from build123d import *

# Parameters (mm, degrees)
CYLINDER055_R       = 2.5
CYLINDER055_DEPTH   = 100
ARRAY001032_Y_COUNT = 6
ARRAY001032_Y_PITCH = 50
BOX030_W            = 3
BOX030_H            = 280
BOX030_DEPTH        = 20
FILLET002_R         = 4


with BuildPart() as horizontal_hole_array006:
    # Cylinder055 → Cylinder055 (new body)
    with BuildSketch(Plane(origin=(-137, -85, -101), x_dir=(0, 0, -1), z_dir=(1, 0, 0))):
        Circle(CYLINDER055_R)
    extrude(amount=CYLINDER055_DEPTH)

    # Array001032 Y: horizontal hole array006 ×6


with BuildPart() as horizontal_hole_array006_1:
    add(horizontal_hole_array006.part)
    with Locations(*[(0, i * ARRAY001032_Y_PITCH, 0) for i in range(1, ARRAY001032_Y_COUNT)]):
        add(horizontal_hole_array006.part)


with BuildPart() as stand_attachment_bottom_plate_cut:
    # Box030 → Box030 (new body)
    with BuildSketch(Plane(origin=(-103, -100, -111), x_dir=(1, 0, 0), z_dir=(0, 0, 1))):
        with Locations((1.5, 140)):
            Rectangle(BOX030_W, BOX030_H)
    extrude(amount=BOX030_DEPTH)

    # Fillet002
    fillet002_edges = [stand_attachment_bottom_plate_cut.edges().sort_by_distance(p)[0] for p in [
        (-101.5, -100, -111),
        (-101.5, -100, -91),
        (-101.5, 180, -111),
        (-101.5, 180, -91),
    ]]
    fillet(fillet002_edges, radius=FILLET002_R)

    # Cut019005: cut horizontal hole array006
    add(horizontal_hole_array006_1.part, mode=Mode.SUBTRACT)


solid = stand_attachment_bottom_plate_cut.part
Verification items for the finished model (mm, model axes). Give positions to 0.01 mm unless a question says otherwise; leave off trailing zeros. Loops run counter-clockwise (first coordinate to the right, second up) from the corner with the lowest first, then second, coordinate; pieces in that order, holes last.
1) Sectioned sample at A-A, the plane z = -101. Enter the section's corners in (x, y).
2) Depth check by flat-ended pin: pin 1 Ø8 at (y, z) = (15, -101) entering from +X; pin 2 Ø3 at (y, z) = (65, -101) entering from -X. Enter the tip coordinate at first touch or a pass-through.
3) Thickness scan on line 1 along Z through (x, y) = (-101.6, -85); line 2 along Y through (x, z) = (-101.35, -107.25); line 3 along Z through (x, y) = (-101.8, 64). Record the ranges inside material, lowest first.
4) Draft check along Z on faces 1 (the cylindrical face through (-101.52, 12.78, -102.15)), 2 (the flat face through (-100, 38, -101)). Enter one of: pulls with the +Z half, pulls with the -Z half, needs draft (parallel to the pull), parting line crosses it, or undercut.
5) Sectioned sample at B-B, the plane x = -101.65. Enter the section's corners in (y, z), then the cut area to 3 significant figures.
6) Sectioned sample at C-C, the plane y = 65. Enter the section's corners in (x, z).
Answers:
1. outline: (-103, -100) - (-100, -100) - (-100, -87.5) - (-103, -87.5) - close; (-103, -82.5) - (-100, -82.5) - (-100, -37.5) - (-103, -37.5) - close; (-103, -32.5) - (-100, -32.5) - (-100, 12.5) - (-103, 12.5) - close; (-103, 17.5) - (-100, 17.5) - (-100, 62.5) - (-103, 62.5) - close; (-103, 67.5) - (-100, 67.5) - (-100, 112.5) - (-103, 112.5) - close; (-103, 117.5) - (-100, 117.5) - (-100, 162.5) - (-103, 162.5) - close; (-103, 167.5) - (-100, 167.5) - (-100, 180) - (-103, 180) - close
2. pin 1: stops at x = -100
2. pin 2: passes through
3. line 1: z = -111 to -103.5, -98.5 to -91
3. line 2: y = -99.99 to 179.99
3. line 3: z = -111 to -103.29, -98.71 to -91
4. face 1: undercut
4. face 2: needs draft
5. outline: (-100, -107) arc R4 ccw to (-96, -111) - (176, -111) arc R4 ccw to (180, -107) - (180, -95) arc R4 ccw to (176, -91) - (-96, -91) arc R4 ccw to (-100, -95) - close; hole circle Ø5 at (-85, -101); hole circle Ø5 at (-35, -101); hole circle Ø5 at (15, -101); hole circle Ø5 at (65, -101); hole circle Ø5 at (115, -101); hole circle Ø5 at (165, -101)
5. area: 5,470 mm2
6. outline: (-103, -111) - (-100, -111) - (-100, -103.5) - (-103, -103.5) - close; (-103, -98.5) - (-100, -98.5) - (-100, -91) - (-103, -91) - close
